from build123d import *

# Parameters (mm, degrees)
SKETCH_1_R             = 62
SKETCH_1_R_2           = 60
EXTRUDE_1_DEPTH        = 3
EXTRUDE_START          = 6
SKETCH_2_R             = 48
EXTRUDE_2_DEPTH        = 6
FILLET_1_R             = 5
CHAMFER_1_SIZE         = 0.5
CHAMFER_2_SIZE         = 0.5
SKETCH_6_R             = 2.2
CUT_EXTRUDE_1_DEPTH    = 6
SKETCH_7_W             = 65
SKETCH_7_H             = 13.477482046
EXTRUDE_3_DEPTH        = 3
SKETCH_11_R            = 1.7
CUT_EXTRUDE_2_DEPTH    = 3
CHAMFER_3_SIZE         = 1
CHAMFER_4_SIZE         = 1
FILLET_2_R             = 3
CHAMFER_5_3_ANGLE      = 291.929687
SKETCH_12_R            = 4
CUT_EXTRUDE_3_DEPTH    = 3
CUT_EXTRUDE_4_DEPTH    = 2
CHAMFER_6_SIZE         = 1
HOLE_WIZARD_M3_1_D     = 2.5
HOLE_WIZARD_M3_1_DEPTH = 7.5
HOLE_WIZARD_M3_1_TIP   = 0.751075774
HOLE_WIZARD_M3_2_D     = 2.5
HOLE_WIZARD_M3_2_DEPTH = 7.5
HOLE_WIZARD_M3_2_TIP   = 0.751075774
SKETCH_21_R            = 2
CUT_EXTRUDE_5_DEPTH    = 13
SKETCH_22_R            = 2
CUT_EXTRUDE_6_DEPTH    = 13
SKETCH_25_R            = 2
CUT_EXTRUDE_8_DEPTH    = 10


with BuildPart() as part:
    # 草图1 → 凸台-拉伸1 (new body)
    with BuildSketch(Plane.XY):
        Circle(SKETCH_1_R)
        Circle(SKETCH_1_R_2, mode=Mode.SUBTRACT)
    extrude(amount=-EXTRUDE_1_DEPTH)

    # 草图2 → 凸台-拉伸2 (add)
    with BuildSketch(Plane.XY.offset(EXTRUDE_START)):
        with BuildLine():
            Line((-32.5, 63), (32.5, 63))
            Line((32.5, 63), (32.5, 52.79914772))
            ThreePointArc((32.5, 52.79914772), (0, -62), (-32.5, 52.79914772))
            Line((-32.5, 52.79914772), (-32.5, 63))
        make_face()
        Circle(SKETCH_2_R, mode=Mode.SUBTRACT)
    extrude(amount=-EXTRUDE_2_DEPTH)

    # 圆角1
    # the kernel refuses this fillet: 5 mm, written as the material it adds along each edge
    with BuildSketch(Plane(origin=(32.5, 52.79914772, 6), x_dir=(0.8403342947446245, -0.5420685132675156, 0), z_dir=(0, 0, -1))) as fillet_1_piece_1:
        with BuildLine():
            CenterArc((2.72541822, -4.998883971), FILLET_1_R, 91.210593649, 55.964843523)
            Line((-1.476253254, -2.288541405), (0, 0))
            ThreePointArc((0, 0), (1.309890927, -0.013838756), (2.619781855, 0))
        make_face()
    extrude(amount=6)
    with BuildSketch(Plane(origin=(-32.5, 52.79914772, 6), x_dir=(-0.840334294744627, -0.5420685132675117, 0), z_dir=(0, 0, -1))) as fillet_1_piece_2:
        with BuildLine():
            CenterArc((2.72541822, 4.998883971), FILLET_1_R, 212.824562828, 55.964843523)
            Line((-1.476253254, 2.288541405), (0, 0))
            ThreePointArc((0, 0), (1.309890927, 0.013838756), (2.619781855, 0))
        make_face()
    extrude(amount=6)

    # 倒角1
    chamfer_1_edges = [part.edges().sort_by_distance(p)[0] for p in [
        (-48, 0, 0),
        (-48, 0, 6),
        (-60, 0, -3),
    ]]
    chamfer(chamfer_1_edges, length=CHAMFER_1_SIZE)

    # 倒角2
    # the kernel refuses this chamfer: 0.5 mm, written as the material it takes off along each edge
    with BuildSketch(Plane(origin=(-32.5, 55.522517954, 0), x_dir=(0, 0, 1), z_dir=(0, 1, 0)), Plane(origin=(32.5, 64.285841494, 0), x_dir=(0, 0, 1), z_dir=(0, -1, 0))) as chamfer_2_piece_1:
        Polygon((CHAMFER_2_SIZE, 0), (0, CHAMFER_2_SIZE), (0, 0), align=None)
    extrude(amount=8.76332354, mode=Mode.SUBTRACT)
    with BuildSketch(Plane(origin=(37.5, 55.522517954, 0), x_dir=(-0.15613015555825177, -0.9877364904291813, 0), z_dir=(0.9877364904291813, -0.15613015555825177, 0))) as chamfer_2_piece_2_section:
        Polygon((5, -CHAMFER_2_SIZE), (5 + CHAMFER_2_SIZE, 0), (5, 0), align=None)
    chamfer_2_piece_2 = revolve(axis=Axis((37.5, 55.522517954, 0), (0, 0, -1)), revolution_arc=81.017652556, mode=Mode.PRIVATE)
    chamfer_2_piece_2 = chamfer_2_piece_2 - Plane(origin=(0, 0, 0), x_dir=(1, 0, 0), z_dir=(0, 0, 1)) * Cylinder(62, 22, mode=Mode.PRIVATE)
    add(chamfer_2_piece_2, mode=Mode.SUBTRACT)
    with BuildSketch(Plane(origin=(-37.5, 55.522517954, 0), x_dir=(1, 0, 0), z_dir=(0, 1, 0))) as chamfer_2_piece_3_section:
        Polygon((5, -CHAMFER_2_SIZE), (5 + CHAMFER_2_SIZE, 0), (5, 0), align=None)
    chamfer_2_piece_3 = revolve(axis=Axis((-37.5, 55.522517954, 0), (0, 0, -1)), revolution_arc=81.017652556, mode=Mode.PRIVATE)
    chamfer_2_piece_3 = chamfer_2_piece_3 - Plane(origin=(0, 0, 0), x_dir=(1, 0, 0), z_dir=(0, 0, 1)) * Cylinder(62, 22, mode=Mode.PRIVATE)
    add(chamfer_2_piece_3, mode=Mode.SUBTRACT)

    # 草图6 → 切除-拉伸1 (cut)
    with BuildSketch(Plane(origin=(0, 0, 0), x_dir=(-1, 0, 0), z_dir=(0, 0, -1))):
        with Locations((-42.877900702, 31.152618372)):
            Circle(SKETCH_6_R)
        with Locations((-53, 0)):
            Circle(SKETCH_6_R)
        with Locations((-42.877900702, -31.152618371)):
            Circle(SKETCH_6_R)
        with Locations((-16.377900702, -50.405995364)):
            Circle(SKETCH_6_R)
        with Locations((16.377900702, -50.405995364)):
            Circle(SKETCH_6_R)
        with Locations((42.877900702, -31.152618371)):
            Circle(SKETCH_6_R)
        with Locations((53, 0)):
            Circle(SKETCH_6_R)
        with Locations((42.877900702, 31.152618372)):
            Circle(SKETCH_6_R)
        with Locations((16.377900702, 50.405995364)):
            Circle(SKETCH_6_R)
        with Locations((-16.377900702, 50.405995364)):
            Circle(SKETCH_6_R)
    extrude(amount=-CUT_EXTRUDE_1_DEPTH, mode=Mode.SUBTRACT)

    # 草图7 → 凸台-拉伸3 (add)
    with BuildSketch(Plane.XY.offset(6)):
        with Locations((0, 62.261258977)):
            Rectangle(SKETCH_7_W, SKETCH_7_H)
    extrude(amount=EXTRUDE_3_DEPTH)

    # 草图11 → 切除-拉伸2 (cut)
    with BuildSketch(Plane.XY.offset(9)):
        with Locations((-29.5, 66)):
            Circle(SKETCH_11_R)
        with Locations((29.5, 66)):
            Circle(SKETCH_11_R)
    extrude(amount=-CUT_EXTRUDE_2_DEPTH, mode=Mode.SUBTRACT)

    # 倒角3
    chamfer_3_edges = [part.edges().sort_by_distance(p)[0] for p in [
        (0, 63, 0),
    ]]
    chamfer(chamfer_3_edges, length=CHAMFER_3_SIZE - 0.0001)  # a hair under: the kernel refuses the full size

    # 倒角4
    chamfer_4_edges = [part.edges().sort_by_distance(p)[0] for p in [
        (0, 55.522517954, 9),
    ]]
    chamfer(chamfer_4_edges, length=CHAMFER_4_SIZE)

    # 圆角2
    fillet_2_edges = [part.edges().sort_by_distance(p)[0] for p in [
        (-32.5, 69, 7.5),
        (32.5, 69, 7.5),
    ]]
    fillet(fillet_2_edges, radius=FILLET_2_R)

    # 倒角5: read off the stored shape, not the designer's step
    # 倒角5 outline → 倒角5 (revolve, cut)
    with BuildSketch(Plane(origin=(37.5, 55.522517954, 0), x_dir=(1, 0, 0), z_dir=(0, -1, 0))):
        Polygon((4.999998721, 9), (4.999998721, 4.999998721), (9, 9), align=None)
    revolve(axis=Axis((37.5, 55.522517954, 0), (0, 0, 1)), mode=Mode.SUBTRACT)

    # Chamfer 5 2 outline → Chamfer 5 2 (revolve, cut)
    with BuildSketch(Plane(origin=(-37.5, 55.522517954, 0), x_dir=(1, 0, 0), z_dir=(0, -1, 0))):
        Polygon((4.99999762, 9), (4.99999762, 4.99999762), (9, 9), align=None)
    revolve(axis=Axis((-37.5, 55.522517954, 0), (0, 0, 1)), mode=Mode.SUBTRACT)

    # Chamfer 5 3 outline → Chamfer 5 3 (revolve, cut)
    with BuildSketch(Plane(origin=(0, 0, 0), x_dir=(-0.5597014925373135, 0.8286942978273132, 0), z_dir=(0.8286942978273132, 0.5597014925373135, 0))):
        Polygon((62, 6), (61, 6), (62, 5), align=None)
    revolve(axis=Axis((0, 0, 0), (0, 0, 1)), revolution_arc=CHAMFER_5_3_ANGLE, mode=Mode.SUBTRACT)

    # 草图12 → 切除-拉伸3 (cut)
    with BuildSketch(Plane.XY.offset(6)):
        with Locations((-16.377900702, 50.405995364)):
            Circle(SKETCH_12_R)
        with Locations((16.377900702, 50.405995364)):
            Circle(SKETCH_12_R)
        with Locations((42.877900702, 31.152618372)):
            Circle(SKETCH_12_R)
        with Locations((53, 0)):
            Circle(SKETCH_12_R)
        with Locations((42.877900702, -31.152618371)):
            Circle(SKETCH_12_R)
        with Locations((16.377900702, -50.405995364)):
            Circle(SKETCH_12_R)
        with Locations((-16.377900702, -50.405995364)):
            Circle(SKETCH_12_R)
        with Locations((-42.877900702, -31.152618371)):
            Circle(SKETCH_12_R)
        with Locations((-53, 0)):
            Circle(SKETCH_12_R)
        with Locations((-42.877900702, 31.152618372)):
            Circle(SKETCH_12_R)
    extrude(amount=-CUT_EXTRUDE_3_DEPTH, mode=Mode.SUBTRACT)

    # 草图14 → 切除-拉伸4 (cut)
    with BuildSketch(Plane(origin=(0, 63, 0), x_dir=(1, 0, 0), z_dir=(0, 1, 0))):
        with BuildLine():
            ThreePointArc((-4.030108666, 3.809429698), (-11.733833556, 7.447967709), (-11.5, -1.068584287))
            ThreePointArc((-11.5, -1.068584287), (0, -4.15), (11.5, -1.068584287))
            ThreePointArc((11.5, -1.068584287), (11.733833556, 7.447967709), (4.030108666, 3.809429698))
            ThreePointArc((4.030108666, 3.809429698), (0, 5.85), (-4.030108666, 3.809429698))
        make_face()
    extrude(amount=-CUT_EXTRUDE_4_DEPTH, mode=Mode.SUBTRACT)

    # 倒角6
    # the kernel refuses this chamfer: 1 mm, written as the material it takes off along each edge
    with BuildSketch(Plane(origin=(18.80558547, 61, -3), x_dir=(0, -1, 0), z_dir=(-1, 0, 0))) as chamfer_6_piece_1:
        Polygon((CHAMFER_6_SIZE, 0), (0, CHAMFER_6_SIZE), (0, 0), align=None)
    extrude(amount=37.61117094, mode=Mode.SUBTRACT)
    with BuildSketch(Plane(origin=(-9, 63, -3.261542732), x_dir=(-0.874686173337968, 0, 0.48468969266055384), z_dir=(-0.48468969266055384, 0, -0.874686173337968))) as chamfer_6_piece_2:
        Polygon((5, -CHAMFER_6_SIZE), (5 + CHAMFER_6_SIZE, 0), (5, 0), align=None)
    revolve(axis=Axis((-9, 63, -3.261542732), (0, 1, 0)), revolution_arc=31.007856081, mode=Mode.SUBTRACT)
    with BuildSketch(Plane(origin=(9, 63, -3.261542732), x_dir=(0.49999999999998873, 0, 0.8660254037844451), z_dir=(-0.8660254037844451, 0, 0.49999999999998873))) as chamfer_6_piece_3:
        Polygon((5, -CHAMFER_6_SIZE), (5 + CHAMFER_6_SIZE, 0), (5, 0), align=None)
    revolve(axis=Axis((9, 63, -3.261542732), (0, 1, 0)), revolution_arc=31.007856081, mode=Mode.SUBTRACT)
    with BuildSketch(Plane(origin=(0, 63, -18.85), x_dir=(-0.500000000000001, 0, 0.8660254037844382), z_dir=(-0.8660254037844382, 0, -0.500000000000001))) as chamfer_6_piece_4:
        Polygon((23, -CHAMFER_6_SIZE), (23 + CHAMFER_6_SIZE, 0), (23, 0), align=None)
    revolve(axis=Axis((0, 63, -18.85), (0, 1, 0)), revolution_arc=60, mode=Mode.SUBTRACT)

    # M3 螺纹孔1
    with Locations(Plane.XY.offset(9)):
        with Locations((-25, 60), (25, 60)):
            Hole(HOLE_WIZARD_M3_1_D / 2, depth=HOLE_WIZARD_M3_1_DEPTH)
            with Locations((0, 0, -(HOLE_WIZARD_M3_1_DEPTH + HOLE_WIZARD_M3_1_TIP / 2))):  # 118° drill point
                Cone(0, HOLE_WIZARD_M3_1_D / 2, HOLE_WIZARD_M3_1_TIP, mode=Mode.SUBTRACT)

    # M3 螺纹孔2
    with Locations(Plane.XY.offset(6)):
        with Locations((0, -53)):
            Hole(HOLE_WIZARD_M3_2_D / 2, depth=HOLE_WIZARD_M3_2_DEPTH)
            with Locations((0, 0, -(HOLE_WIZARD_M3_2_DEPTH + HOLE_WIZARD_M3_2_TIP / 2))):  # 118° drill point
                Cone(0, HOLE_WIZARD_M3_2_D / 2, HOLE_WIZARD_M3_2_TIP, mode=Mode.SUBTRACT)

    # 草图21 → 切除-拉伸5 (cut)
    with BuildSketch(Plane.XY.offset(6)):
        with Locations((-4.968742047, -51.94347744)):
            Circle(SKETCH_21_R)
    extrude(amount=-CUT_EXTRUDE_5_DEPTH, mode=Mode.SUBTRACT)

    # 草图22 → 切除-拉伸6 (cut)
    with BuildSketch(Plane.XY.offset(6)):
        with Locations((-47.468742054, 21.668681868)):
            Circle(SKETCH_22_R)
    extrude(amount=-CUT_EXTRUDE_6_DEPTH, mode=Mode.SUBTRACT)

    # 草图25 → 切除-拉伸8 (cut)
    with BuildSketch(Plane.XY.offset(6)):
        with Locations((47.468742054, 21.668681868)):
            Circle(SKETCH_25_R)
        with Locations((4.968742047, -51.94347744)):
            Circle(SKETCH_25_R)
    extrude(amount=-CUT_EXTRUDE_8_DEPTH, mode=Mode.SUBTRACT)


solid = part.part
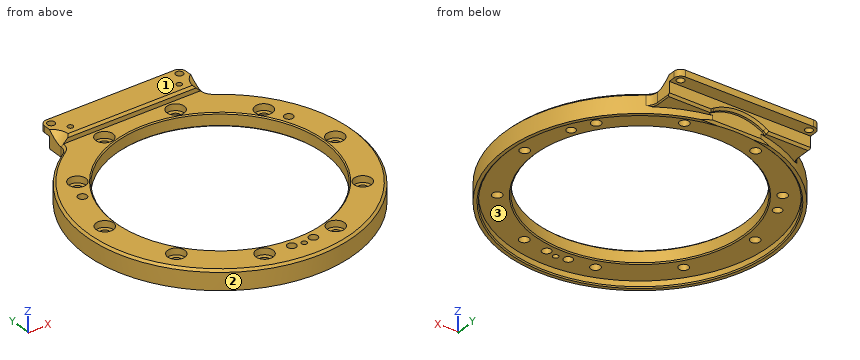
Geometry: final body of the model. Coordinates: model frame, mm. Face numbers are marked on the shaded views. Give positions to 0.01 mm unless a question says otherwise; leave off trailing zeros. Answer in a Markdown table with one row per item. Add a question column.
(1) Ray query, line 1 (X direction, y = 60, z = 4.5); line 2 (X direction, y = 66, z = 7.65); line 3 (Y direction, x = 44, z = 1.25). Return the intervals inside material, ascending.
(2) Mould query, pull axis Y, two halves, no side actions, for the marked faces 1, 2 and 3. Classes: +Y half, -Y half, draft (parallel to the pull), parting line (faces both ways), or undercut.
(3) First-contact query: pin 1 (0.6 mm diameter, centred on x = -6, z = 7, fed in from -Y); pin 2 (9 mm diameter, centred on x = -16.38, y = 50.41, fed in from +Z); pin 3 (4 mm diameter, centred on y = -13.5, z = 4, fed in from +X). Flat tips, straight axial feed; report the tip coordinate or a pass-through.
Result set:
| question | item | result |
|---|---|---|
| 1 | line 1 | x = -32.5 to -26.25, -23.75 to 23.75, 26.25 to 32.5 |
| 1 | line 2 | x = -32.5 to -31.2, -27.8 to 27.8, 31.2 to 32.5 |
| 1 | line 3 | y = -43.68 to -33.04, -29.26 to -19.18, 19.18 to 29.26, 33.04 to 43.68 |
| 2 | face 1 | draft |
| 2 | face 2 | parting line |
| 2 | face 3 | undercut |
| 3 | pin 1 | stops at y = 55.52 |
| 3 | pin 2 | stops at z = 6 |
| 3 | pin 3 | stops at x = 60.92 |
